Design review of the part shown in the three views and the two pictorial views. Dimensions are in mm from the part's minimum x, y and z. Give positions to 0.01 mm unless a question says otherwise; leave off trailing zeros. Loops run counter-clockwise (first coordinate to the right, second up) from the corner with the lowest first, then second, coordinate; pieces in that order, holes last. Notation, with made-up numbers: (43.5, -7) - (93.5, -7) arc R23 ccw to (93.5, 22) - close; hole circle Ø7 at (-3.75, 26). An arc over 180 degrees is marked (long way). Use CSV: the item, a comma, the result in double quotes. Start each with the question number.
1. Take a section at A-A on x = 0.4. Give the boundary of the cut face in (y, z), plus the area to 3 significant figures.
2. For pin 1 (1 mm diameter, centred on x = 1.5, y = 11.5, fed in from +Z), flat-tipped, find the tip position at first contact; note if it passes through.
3. Take a section at B-B on y = 4. Give the boundary of the cut face in (x, z), plus the area to 3 significant figures.
4. Wall thickness on line 1 (Y direction, x = 1.6, z = 1.6); line 2 (Z direction, x = 1, y = 30.5); line 3 (Z direction, x = 1.8, y = 15): over which ranges is each line inside the solid? List them lowest first.
5. Take a section at C-C on z = 0.3. Give the boundary of the cut face in (x, y), plus the area to 3 significant figures.
6. Mouldability with a two-part tool opening along Y and no side actions: class the marked faces 1, 2 and 3 as pulls with the +Y half, pulls with the -Y half, needs draft (parallel to the pull), parting line crosses it, or undercut.
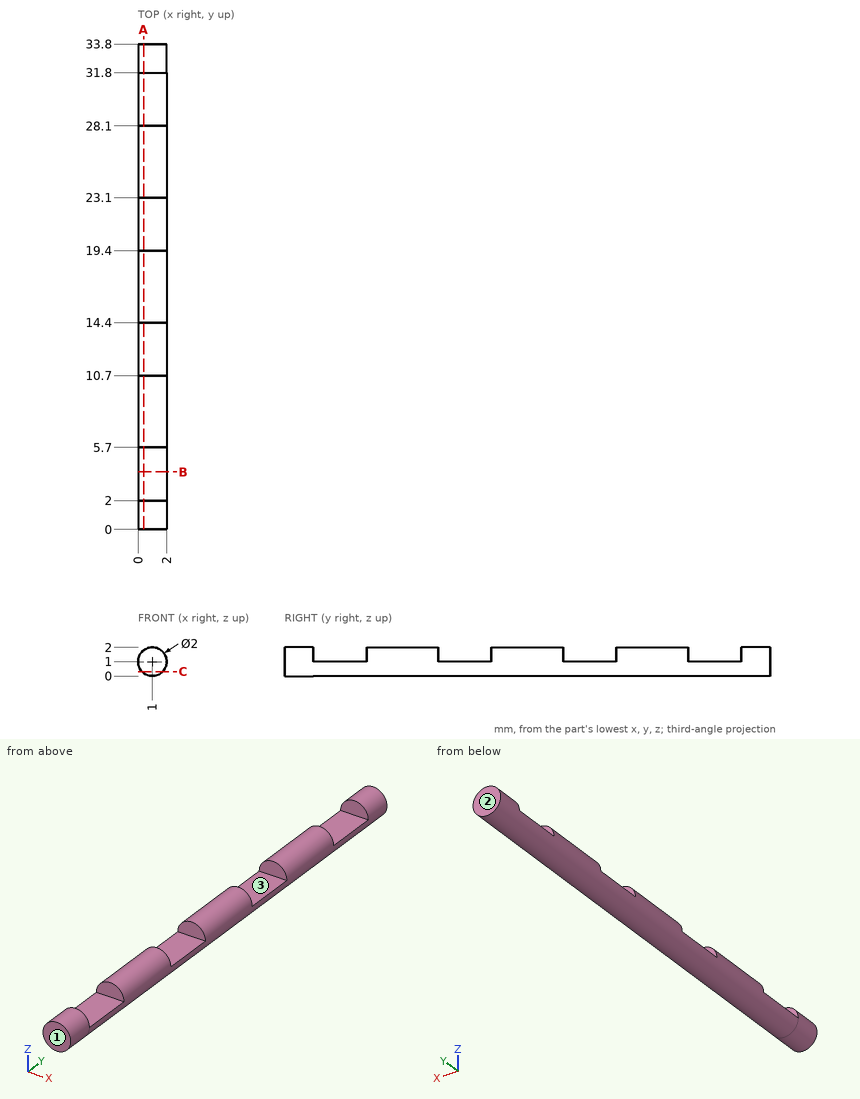
Check result:
1,outline,"(0, 0.2) - (33.8, 0.2) - (33.8, 1.8) - (31.8, 1.8) - (31.8, 1) - (28.1, 1) - (28.1, 1.8) - (23.1, 1.8) - (23.1, 1) - (19.4, 1) - (19.4, 1.8) - (14.4, 1.8) - (14.4, 1) - (10.7, 1) - (10.7, 1.8) - (5.7, 1.8) - (5.7, 1) - (2, 1) - (2, 1.8) - (0, 1.8) - close"
1,area,"42.2 mm²"
2,pin 1,"stops at z = 1"
3,outline,"(0, 1) arc R1 ccw to (2, 1) - close"
3,area,"1.57 mm²"
4,line 1,"y = 0 to 2, 5.7 to 10.7, 14.4 to 19.4, 23.1 to 28.1, 31.8 to 33.8"
4,line 2,"z = 0 to 1"
4,line 3,"z = 0.4 to 1.6"
5,outline,"(0.29, 0) - (1.71, 0) - (1.71, 33.8) - (0.29, 33.8) - close"
5,area,"48.3 mm²"
6,face 1,"pulls with the -Y half"
6,face 2,"pulls with the +Y half"
6,face 3,"undercut"
